from build123d import *

# Parameters (mm, degrees)
SKETCH2_W                   = 101.6
SKETCH2_H                   = 101.6
SKETCH2_R                   = 4.7625
BOSS_EXTRUDE1_DEPTH         = 19.05
TAP_DRILL_FOR_M3X0_5_TAP1_D = 2.5


with BuildPart() as part:
    # Sketch2 → Boss-Extrude1 (new body)
    with BuildSketch(Plane(origin=(0, 0, 0), x_dir=(1, 0, 0), z_dir=(0, 1, 0))):
        with Locations((30.8, -30.8)):
            Rectangle(SKETCH2_W, SKETCH2_H)
        with Locations(Location((70.710678119, -70.710678119, 0), (0, 0, 270))):
            Circle(SKETCH2_R, mode=Mode.SUBTRACT)
        with BuildLine():
            ThreePointArc((-3.18, -3.18), (-6.36, 0), (-3.18, 3.18))
            ThreePointArc((-3.18, 3.18), (0, 6.36), (3.18, 3.18))
            ThreePointArc((3.18, 3.18), (6.36, 0), (3.18, -3.18))
            ThreePointArc((3.18, -3.18), (0, -6.36), (-3.18, -3.18))
        make_face(mode=Mode.SUBTRACT)
    extrude(amount=-BOSS_EXTRUDE1_DEPTH)

    # Tap Drill for M3x0.5 Tap1 (through all)
    with Locations(Plane(origin=(0, 0, -10), x_dir=(0, 0, 1), z_dir=(0, 1, 0))):
        with Locations((0, 0), (10, 10), (20, 0), (10, -10)):
            Hole(TAP_DRILL_FOR_M3X0_5_TAP1_D / 2)


solid = part.part
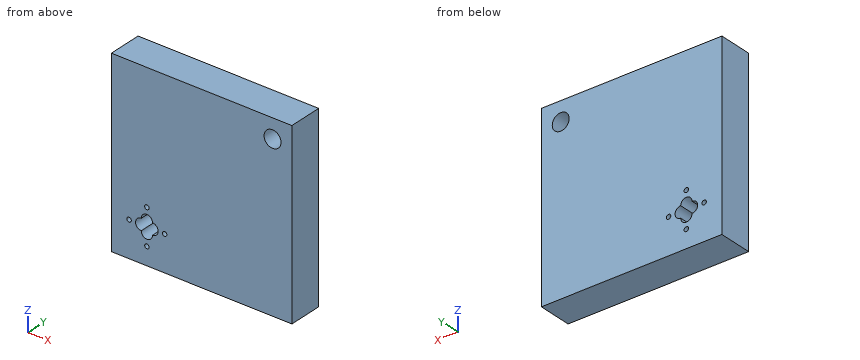
Work out the finished part from the listing and answer in its coordinate system (mm). Give positions to 0.01 mm unless a question says otherwise; leave off trailing zeros. Write each loop counter-clockwise with the first axis right and the second up, starting at its lowest first coordinate (ties: lowest second). Pieces come first, ordered by that corner, then holes.
Q1. The part is cut by section A-A on x = -10. Give the vertices of the cut face in (y, z).
Answer:
outline: (-19.05, -20) - (0, -20) - (0, -1.25) - (-19.05, -1.25) - close; (-19.05, 1.25) - (0, 1.25) - (0, 81.6) - (-19.05, 81.6) - close
Q2. The part is cut by section B-B on z = -10. Give the vertices of the cut face in (x, y), and give its area (3 significant figures).
Answer:
outline: (-20, -19.05) - (-1.25, -19.05) - (-1.25, 0) - (-20, 0) - close; (1.25, -19.05) - (81.6, -19.05) - (81.6, 0) - (1.25, 0) - close
area: 1,890 mm2
Q3. The part is cut by section C-C on y = -1.5. State how many separate pieces and enclosed holes the cut face has, and give its area (3 significant figures).
Answer:
separate pieces: 1
enclosed holes: 6
area: 10,100 mm2
Q4. Straight lines are drawn through the part: L1, parallel to X at y = -8, z = 0; L2, parallel to X at y = -13.25, z = -10; L3, parallel to Z at x = 5, y = -7.25. For each, find the intervals that lie inside material, in ascending order.
Answer:
L1: x = -20 to -11.25, -8.75 to -6.36, 6.36 to 8.75, 11.25 to 81.6
L2: x = -20 to -1.25, 1.25 to 81.6
L3: z = -20 to -2.61, 2.61 to 81.6
